Autodesk Fusion 360 part; units mm, degrees
sketch "Boceto1" plane through (0, 0, 0) normal (0, 1, 0) x (1, 0, 0)
  circle A0 centre (0, 0) radius 12.5
  spline S0 degree 5 poles (0.0283, -12.5) (0.331, -13.0785) (0.9099, -14.2374) (1.6984, -15.9815) (2.5873, -18.3184) (3.4097, -21.2601) (3.9181, -24.224) (4.0879, -27.2119) (3.9073, -30.2248) (3.3923, -33.2613) (2.5689, -36.3197) (1.6843, -38.7825) (0.9018, -40.638) (0.3281, -41.8787) (0.0283, -42.5) knots 0 0 0 0 0 0 0.1 0.2 0.3 0.4 0.5 0.6 0.7 0.8 0.9 1 1 1 1 1 1
  spline S1 degree 5 poles (10.8394, -6.2255) (11.4918, -6.2526) (12.7849, -6.3307) (14.6896, -6.5199) (17.1579, -6.9185) (20.1166, -7.6771) (22.9377, -8.7188) (25.6102, -10.0658) (28.1291, -11.7286) (30.5013, -13.6929) (32.7383, -15.9351) (34.4288, -17.9326) (35.6444, -19.538) (36.4321, -20.6552) (36.8202, -21.2255) knots 0 0 0 0 0 0 0.1 0.2 0.3 0.4 0.5 0.6 0.7 0.8 0.9 1 1 1 1 1 1
  spline S2 degree 5 poles (10.8112, 6.2745) (11.1608, 6.8259) (11.875, 7.9067) (12.9912, 9.4616) (14.5705, 11.3999) (16.7069, 13.5829) (19.0195, 15.5052) (21.5223, 17.1462) (24.2218, 18.4962) (27.109, 19.5684) (30.1693, 20.3846) (32.7445, 20.8499) (34.7427, 21.1) (36.104, 21.2235) (36.7919, 21.2745) knots 0 0 0 0 0 0 0.1 0.2 0.3 0.4 0.5 0.6 0.7 0.8 0.9 1 1 1 1 1 1
  spline S3 degree 5 poles (-0.0283, 12.5) (-0.331, 13.0785) (-0.9099, 14.2374) (-1.6984, 15.9815) (-2.5873, 18.3184) (-3.4097, 21.2601) (-3.9181, 24.224) (-4.0879, 27.2119) (-3.9073, 30.2248) (-3.3923, 33.2613) (-2.5689, 36.3197) (-1.6843, 38.7825) (-0.9018, 40.638) (-0.3281, 41.8787) (-0.0283, 42.5) knots 0 0 0 0 0 0 0.1 0.2 0.3 0.4 0.5 0.6 0.7 0.8 0.9 1 1 1 1 1 1
  spline S4 degree 5 poles (-10.8394, 6.2255) (-11.4918, 6.2526) (-12.7849, 6.3307) (-14.6896, 6.5199) (-17.1579, 6.9185) (-20.1166, 7.6771) (-22.9377, 8.7188) (-25.6102, 10.0658) (-28.1291, 11.7286) (-30.5013, 13.6929) (-32.7383, 15.9351) (-34.4288, 17.9326) (-35.6444, 19.538) (-36.4321, 20.6552) (-36.8202, 21.2255) knots 0 0 0 0 0 0 0.1 0.2 0.3 0.4 0.5 0.6 0.7 0.8 0.9 1 1 1 1 1 1
  spline S5 degree 5 poles (-10.8112, -6.2745) (-11.1608, -6.8259) (-11.875, -7.9067) (-12.9912, -9.4616) (-14.5705, -11.3999) (-16.7069, -13.5829) (-19.0195, -15.5052) (-21.5223, -17.1462) (-24.2218, -18.4962) (-27.109, -19.5684) (-30.1693, -20.3846) (-32.7445, -20.8499) (-34.7427, -21.1) (-36.104, -21.2235) (-36.7919, -21.2745) knots 0 0 0 0 0 0 0.1 0.2 0.3 0.4 0.5 0.6 0.7 0.8 0.9 1 1 1 1 1 1
  spline S6 degree 3 poles (2.6863, -11.1089) (4.8889, -15.3178) (6.376, -19.6566) (6.8447, -24.1702) (7.2296, -27.8773) (6.8659, -31.6563) (5.8959, -35.3638) (5.1552, -38.1952) (4.0833, -41.0001) (2.7301, -43.8039) knots 0 0 0 0 0.408399 0.408399 0.408399 0.743829 0.743829 0.743829 1 1 1 1
  spline S7 degree 3 poles (10.9638, -3.2281) (15.7101, -3.425) (20.2111, -4.3065) (24.3543, -6.1574) (27.7573, -7.6776) (30.8481, -9.8821) (33.5739, -12.5759) (35.6556, -14.6331) (37.5487, -16.9638) (39.3004, -19.5377) knots 0 0 0 0 0.408399 0.408399 0.408399 0.743829 0.743829 0.743829 1 1 1 1
  spline S8 degree 3 poles (8.2775, 7.8809) (10.8212, 11.8928) (13.8351, 15.3501) (17.5096, 18.0128) (20.5276, 20.1997) (23.9822, 21.7741) (27.678, 22.7879) (30.5004, 23.5621) (33.4655, 24.0362) (36.5703, 24.2663) knots 0 0 0 0 0.408399 0.408399 0.408399 0.743829 0.743829 0.743829 1 1 1 1
  spline S9 degree 3 poles (-2.6863, 11.1089) (-4.8889, 15.3178) (-6.376, 19.6566) (-6.8447, 24.1702) (-7.2296, 27.8773) (-6.8659, 31.6563) (-5.8959, 35.3638) (-5.1552, 38.1952) (-4.0833, 41.0001) (-2.7301, 43.8039) knots 0 0 0 0 0.408399 0.408399 0.408399 0.743829 0.743829 0.743829 1 1 1 1
  spline S10 degree 3 poles (-10.9638, 3.2281) (-15.7101, 3.425) (-20.2111, 4.3065) (-24.3543, 6.1574) (-27.7573, 7.6776) (-30.8481, 9.8821) (-33.5739, 12.5759) (-35.6556, 14.6331) (-37.5487, 16.9638) (-39.3004, 19.5377) knots 0 0 0 0 0.408399 0.408399 0.408399 0.743829 0.743829 0.743829 1 1 1 1
  spline S11 degree 3 poles (-8.2775, -7.8809) (-10.8212, -11.8928) (-13.8351, -15.3501) (-17.5096, -18.0128) (-20.5276, -20.1997) (-23.9822, -21.7741) (-27.678, -22.7879) (-30.5004, -23.5621) (-33.4655, -24.0362) (-36.5703, -24.2663) knots 0 0 0 0 0.408399 0.408399 0.408399 0.743829 0.743829 0.743829 1 1 1 1
  line L0 (0.0283, -42.5) -> (2.7301, -43.8039)
  line L1 (36.8202, -21.2255) -> (39.3004, -19.5377)
  line L2 (-36.5703, -24.2663) -> (-36.7919, -21.2745)
  line L3 (-39.3004, 19.5377) -> (-36.8202, 21.2255)
  line L4 (-2.7301, 43.8039) -> (-0.0283, 42.5)
  line L5 (36.5703, 24.2663) -> (36.7919, 21.2745)
  point P0 (4, -27)
  point P1 (25.3827, -10.0359)
  point P2 (21.3827, 16.9641)
  point P3 (-4, 27)
  point P4 (-25.3827, 10.0359)
  point P5 (-21.3827, -16.9641)
  dimension "d1" = 25
  dimension "d5" = -3
extrude "Extruir1" add sketch "Boceto1" along normal blind 50
sketch "Boceto2" plane through (0, 0, 0) normal (0, -1, 0) x (1, 0, 0)
  arc A0 (-0.0283, -12.5) -> (8.8761, -8.8014) centre (0, 0) ccw
  spline S0 degree 3 poles (8.8761, -8.8014) (11.2912, -12.4227) (14.1192, -15.556) (17.5096, -18.0128) (20.5276, -20.1997) (23.9822, -21.7741) (27.678, -22.7879) (30.5004, -23.5621) (33.4655, -24.0362) (36.5703, -24.2663) knots 0.031578 0.031578 0.031578 0.031578 0.408399 0.408399 0.408399 0.743829 0.743829 0.743829 1 1 1 1
  line L0 (36.5703, -24.2663) -> (36.7919, -21.2745)
  spline S1 degree 5 poles (10.8112, -6.2745) (11.1608, -6.8259) (11.875, -7.9067) (12.9912, -9.4616) (14.5705, -11.3999) (16.7069, -13.5829) (19.0195, -15.5052) (21.5223, -17.1462) (24.2218, -18.4962) (27.109, -19.5684) (30.1693, -20.3846) (32.7445, -20.8499) (34.7427, -21.1) (36.104, -21.2235) (36.7919, -21.2745) knots 0 0 0 0 0 0 0.1 0.2 0.3 0.4 0.5 0.6 0.7 0.8 0.9 1 1 1 1 1 1
  arc A1 (10.8112, -6.2745) -> (12.0603, 3.2862) centre (0, 0) ccw
  spline S2 degree 3 poles (12.0603, 3.2862) (16.404, 3.5671) (20.5315, 4.4496) (24.3543, 6.1574) (27.7573, 7.6776) (30.8481, 9.8821) (33.5739, 12.5759) (35.6556, 14.6331) (37.5487, 16.9638) (39.3004, 19.5377) knots 0.031578 0.031578 0.031578 0.031578 0.408399 0.408399 0.408399 0.743829 0.743829 0.743829 1 1 1 1
  line L1 (39.3004, 19.5377) -> (36.8202, 21.2255)
  spline S3 degree 5 poles (10.8394, 6.2255) (11.4918, 6.2526) (12.7849, 6.3307) (14.6896, 6.5199) (17.1579, 6.9185) (20.1166, 7.6771) (22.9377, 8.7188) (25.6102, 10.0658) (28.1291, 11.7286) (30.5013, 13.6929) (32.7383, 15.9351) (34.4288, 17.9326) (35.6444, 19.538) (36.4321, 20.6552) (36.8202, 21.2255) knots 0 0 0 0 0 0 0.1 0.2 0.3 0.4 0.5 0.6 0.7 0.8 0.9 1 1 1 1 1 1
  arc A2 (10.8394, 6.2255) -> (3.1842, 12.0876) centre (0, 0) ccw
  spline S4 degree 3 poles (3.1842, 12.0876) (5.1128, 15.9898) (6.4123, 20.0056) (6.8447, 24.1702) (7.2296, 27.8773) (6.8659, 31.6563) (5.8959, 35.3638) (5.1552, 38.1952) (4.0833, 41.0001) (2.7301, 43.8039) knots 0.031578 0.031578 0.031578 0.031578 0.408399 0.408399 0.408399 0.743829 0.743829 0.743829 1 1 1 1
  line L2 (2.7301, 43.8039) -> (0.0283, 42.5)
  spline S5 degree 5 poles (0.0283, 12.5) (0.331, 13.0785) (0.9099, 14.2374) (1.6984, 15.9815) (2.5873, 18.3184) (3.4097, 21.2601) (3.9181, 24.224) (4.0879, 27.2119) (3.9073, 30.2248) (3.3923, 33.2613) (2.5689, 36.3197) (1.6843, 38.7825) (0.9018, 40.638) (0.3281, 41.8787) (0.0283, 42.5) knots 0 0 0 0 0 0 0.1 0.2 0.3 0.4 0.5 0.6 0.7 0.8 0.9 1 1 1 1 1 1
  arc A3 (0.0283, 12.5) -> (-8.8761, 8.8014) centre (0, 0) ccw
  spline S6 degree 3 poles (-8.8761, 8.8014) (-11.2912, 12.4227) (-14.1192, 15.556) (-17.5096, 18.0128) (-20.5276, 20.1997) (-23.9822, 21.7741) (-27.678, 22.7879) (-30.5004, 23.5621) (-33.4655, 24.0362) (-36.5703, 24.2663) knots 0.031578 0.031578 0.031578 0.031578 0.408399 0.408399 0.408399 0.743829 0.743829 0.743829 1 1 1 1
  line L3 (-36.5703, 24.2663) -> (-36.7919, 21.2745)
  spline S7 degree 5 poles (-10.8112, 6.2745) (-11.1608, 6.8259) (-11.875, 7.9067) (-12.9912, 9.4616) (-14.5705, 11.3999) (-16.7069, 13.5829) (-19.0195, 15.5052) (-21.5223, 17.1462) (-24.2218, 18.4962) (-27.109, 19.5684) (-30.1693, 20.3846) (-32.7445, 20.8499) (-34.7427, 21.1) (-36.104, 21.2235) (-36.7919, 21.2745) knots 0 0 0 0 0 0 0.1 0.2 0.3 0.4 0.5 0.6 0.7 0.8 0.9 1 1 1 1 1 1
  arc A4 (-10.8112, 6.2745) -> (-12.0603, -3.2862) centre (0, 0) ccw
  spline S8 degree 3 poles (-12.0603, -3.2862) (-16.404, -3.5671) (-20.5315, -4.4496) (-24.3543, -6.1574) (-27.7573, -7.6776) (-30.8481, -9.8821) (-33.5739, -12.5759) (-35.6556, -14.6331) (-37.5487, -16.9638) (-39.3004, -19.5377) knots 0.031578 0.031578 0.031578 0.031578 0.408399 0.408399 0.408399 0.743829 0.743829 0.743829 1 1 1 1
  line L4 (-39.3004, -19.5377) -> (-36.8202, -21.2255)
  spline S9 degree 5 poles (-10.8394, -6.2255) (-11.4918, -6.2526) (-12.7849, -6.3307) (-14.6896, -6.5199) (-17.1579, -6.9185) (-20.1166, -7.6771) (-22.9377, -8.7188) (-25.6102, -10.0658) (-28.1291, -11.7286) (-30.5013, -13.6929) (-32.7383, -15.9351) (-34.4288, -17.9326) (-35.6444, -19.538) (-36.4321, -20.6552) (-36.8202, -21.2255) knots 0 0 0 0 0 0 0.1 0.2 0.3 0.4 0.5 0.6 0.7 0.8 0.9 1 1 1 1 1 1
  arc A5 (-10.8394, -6.2255) -> (-3.1842, -12.0876) centre (0, 0) ccw
  spline S10 degree 3 poles (-3.1842, -12.0876) (-5.1128, -15.9898) (-6.4123, -20.0056) (-6.8447, -24.1702) (-7.2296, -27.8773) (-6.8659, -31.6563) (-5.8959, -35.3638) (-5.1552, -38.1952) (-4.0833, -41.0001) (-2.7301, -43.8039) knots 0.031578 0.031578 0.031578 0.031578 0.408399 0.408399 0.408399 0.743829 0.743829 0.743829 1 1 1 1
  line L5 (-2.7301, -43.8039) -> (-0.0283, -42.5)
  spline S11 degree 5 poles (-0.0283, -12.5) (-0.331, -13.0785) (-0.9099, -14.2374) (-1.6984, -15.9815) (-2.5873, -18.3184) (-3.4097, -21.2601) (-3.9181, -24.224) (-4.0879, -27.2119) (-3.9073, -30.2248) (-3.3923, -33.2613) (-2.5689, -36.3197) (-1.6843, -38.7825) (-0.9018, -40.638) (-0.3281, -41.8787) (-0.0283, -42.5) knots 0 0 0 0 0 0 0.1 0.2 0.3 0.4 0.5 0.6 0.7 0.8 0.9 1 1 1 1 1 1
  line L6 (0, 0) -> (-2.5, 0)
  line L7 (-2.5, 0) -> (-2.5, 1.5)
  line L8 (-2.5, 1.5) -> (2.5, 1.5)
  line L9 (2.5, 1.5) -> (2.5, -1.5)
  line L10 (2.5, -1.5) -> (-2.5, -1.5)
  line L11 (-2.5, -1.5) -> (-2.5, 0)
  line L12 (-3.5, -2.5) -> (-3.5, 2.5)
  line L13 (-3.5, 2.5) -> (3.5, 2.5)
  line L14 (3.5, 2.5) -> (3.5, -2.5)
  line L15 (3.5, -2.5) -> (-3.5, -2.5)
  dimension "d10" = 2.5
  dimension "d11" = 1.5
  dimension "d12" = 5
  dimension "d13" = 3
extrude "Extruir2" add sketch "Boceto2" along normal blind 6 contours L12 L13 L14 L15
sketch "Boceto3" plane through (0, 0, 0) normal (0, 1, 0) x (1, 0, 0)
  line L0 (0, 0) -> (0, -2.9052)
The listing builds one solid part. Answer for the finished solid, in the listing's coordinates (mm). A direction names the side the tool comes from. Round coordinates to 2 decimals unless told otherwise and drop trailing zeros. Loops run counter-clockwise (first coordinate to the right, second up) from the corner with the lowest first, then second, coordinate; pieces in that order, holes last. Notation, with made-up numbers: (71, 81) - (100, 81) arc R33 ccw to (100, 110) - close; hole circle Ø2 at (83.25, -26). An arc over 180 degrees is marked (long way). Use one line per item in the form item = value. Start each with the question number.
1. The part is cut by section A-A on y = -2. Determine the outline of the cut face in (x, z), then the cut area to 3 significant figures.
2. A tool of negligible diameter and unlimited length cuts with its end or side. For faces 5 (the face through (0, -3, 2.5)), 6 (the face through (0, -3, 1.5)), 7 (the face through (0, -3, -2.5)), from which of +Z, -Z, +X, -X, +Y, -Y can it reach the whole face along a straight path? Write none if from no direction.
3. Given pin 1 Ø12 at (y, z) = (7, 12.5) entering from +X; pin 2 Ø3 at (y, z) = (8.5, 20.5) entering from +X; pin 3 Ø3 at (x, y) = (-1.5, -4) entering from +Z; pin 4 Ø2 at (x, z) = (9, -11.5) entering from +Y, each flat-ended and moving along its own axis, determine where each tip first touches the part or whether it passes through.
4. The part is cut by section B-B on z = 16.5. Give the number of separate pieces and of enclosed holes in the cut face, then the cut area to 3 significant figures.
5. Consider line 1 (X direction, y = 45, z = 14.5); line 2 (X direction, y = 5, z = -16.5); line 3 (Z direction, x = 34, y = 35.5). Determine where each line is inside the solid, lowest interval first. Write a range as [from, to].
6. For a pull along X with two mould halves and no side action, classify faces 1 (the face through (38.043, 24.65, 20.393)), 2 (the face through (0, -6, 2)), 3 (the face through (-3.5, -3, 0)), 4 (the face through (0, 0, 0)) as pulls with the +X half, pulls with the -X half, needs draft (parallel to the pull), parting line crosses it, or undercut.
Geometry check:
q1.outline = (-3.5, -2.5) - (3.5, -2.5) - (3.5, 2.5) - (-3.5, 2.5) - close; hole (-2.5, -1.5) - (2.5, -1.5) - (2.5, 1.5) - (-2.5, 1.5) - close
q1.area = 20.0 mm^2
q2.face_5 = +Z, +X, -X, -Y
q2.face_6 = -Y
q2.face_7 = -Z, +X, -X, -Y
q3.pin_1 = 38.58
q3.pin_2 = 39.3
q3.pin_3 = 2.5
q3.pin_4 = through
q4.separate_pieces = 3
q4.enclosed_holes = 0
q4.area = 608 mm^2
q5.line_1 = [-17.87, -13.45], [1.01, 4.29], [31.25, 35.4]
q5.line_2 = [-37.07, -33.16], [-5.07, -1.86], [15.59, 20.62]
q5.line_3 = [-24.01, -20.99], [13, 17.48]
q6.face_1 = pulls with the +X half
q6.face_2 = needs draft
q6.face_3 = pulls with the -X half
q6.face_4 = undercut
